Here's how the part is built. I have some questions about the finished solid (model axes, mm). Round coordinates to 2 decimals unless told otherwise and drop trailing zeros. Write each loop counter-clockwise with the first axis right and the second up, starting at its lowest first coordinate (ties: lowest second). Pieces come first, ordered by that corner, then holes. Notation, with made-up numbers: M 28,35.5 L 64,35.5 A13 ccw 64,47.5 Z; hole C 72,35 d4. An arc over 180 degrees is marked long. Write item = value, one per line. Start each with the question number.
(1) I want a section at A-A (x = 4.75). List the corners of the cut face in (y, z) for me, and give its area (3 significant figures).
(2) I want a section at C-C (x = 8). List the corners of the cut face in (y, z) for me.
(3) I want a section at B-B (y = 2.25). List the corners of the cut face in (x, z) for me.
(4) I need wall thicknesses on line 1 along X through (y, z) = (6, 0.05); line 2 along X through (y, z) = (5.5, 0.05). Which ranges of each line are inside material? Lowest first, please.
(5) I want a section at D-D (y = 5.75). List the corners of the cut face in (x, z) for me, and give its area (3 significant figures).
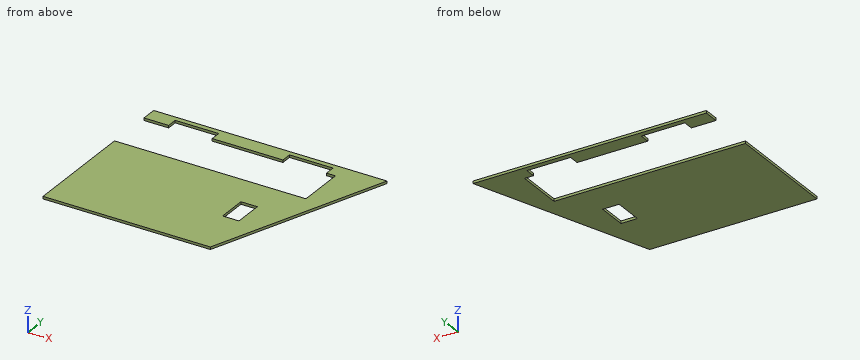
Solid Edge part; units mm, degrees
sketch "Sketch1" plane through (0, 0, 0) normal (0, 0, 1) x (1, 0, 0)
  line L0 (-0.1, 4.6) -> (-0.1, 0)
  line L1 (6.623, 0) -> (-0.1, 0)
  line L2 (6.623, 0) -> (9.2723, 7.1216)
  line L3 (9.2723, 7.1216) -> (-0.1, 7.1216)
  line L4 (-0.1, 7.1216) -> (-0.1, 6.5)
  line L5 (7.59, 6.5) -> (-0.1, 6.5)
  line L6 (7.59, 4.6) -> (7.59, 6.5)
  line L7 (-0.1, 4.6) -> (7.59, 4.6)
  dimension "D1" = 0.1
  dimension "D2" = 0.1
  dimension "D3" = 7.59
extrude "Protrusion1" add sketch "Sketch1" along normal blind 0.1
sketch "Sketch2" plane through (4.6037, 3.5608, 0.1) normal (0, 0, 1) x (-1, 0, 0)
  line L0 (-1.8763, 0.3108) -> (-1.2163, 0.3108)
  line L1 (-1.2163, 0.3108) -> (-1.2163, 1.4908)
  line L2 (-1.2163, 1.4908) -> (-1.8763, 1.4908)
  line L3 (-1.8763, 1.4908) -> (-1.8763, 0.3108)
  dimension "D1" = 1.2163
  dimension "D2" = 1.8763
  dimension "D3" = 1.2163
extrude "Cutout1" cut sketch "Sketch2" against normal through all
sketch "Sketch3" plane through (4.5862, 3.5608, 0.1) normal (0, 0, 1) x (-1, 0, 0)
  line L0 (-0.8938, -2.9392) -> (-2.6438, -2.9392)
  line L1 (-2.6438, -3.3592) -> (-2.6438, -2.9392)
  line L2 (-2.6438, -3.3592) -> (-0.8938, -3.3592)
  line L3 (-0.8938, -2.9392) -> (-0.8938, -3.3592)
  line L4 (1.9462, -2.9392) -> (1.9462, -3.3592)
  line L5 (1.9462, -3.3592) -> (3.6962, -3.3592)
  line L6 (3.6962, -3.3592) -> (3.6962, -2.9392)
  line L7 (3.6962, -2.9392) -> (1.9462, -2.9392)
extrude "Cutout2" cut sketch "Sketch3" against normal through all
Returned:
q1.outline = M 0,0 L 4.6,0 L 4.6,0.1 L 0,0.1 Z; M 6.5,0 L 7.12,0 L 7.12,0.1 L 6.5,0.1 Z
q1.area = 0.522 mm²
q2.outline = M 3.7,0 L 7.12,0 L 7.12,0.1 L 3.7,0.1 Z
q3.outline = M -0.1,0 L 5.82,0 L 5.82,0.1 L -0.1,0.1 Z; M 6.48,0 L 7.46,0 L 7.46,0.1 L 6.48,0.1 Z
q4.line_1 = 7.59 to 8.86
q4.line_2 = 7.59 to 8.67
q5.outline = M 7.59,0 L 8.76,0 L 8.76,0.1 L 7.59,0.1 Z
q5.area = 0.117 mm²
